from build123d import *

# Parameters (mm, degrees)
SKETCH2_W               = 58.32
SKETCH2_H               = 25.24
BOSS_EXTRUDE1_DEPTH     = 5
SKETCH1_R               = 2.25
SKETCH1_R_2             = 2.250000002
SKETCH1_R_3             = 2.250018527
CUT_EXTRUDE1_DEPTH      = 6
CUT_EXTRUDE1_DEPTH_BACK = 6
SKETCH3_W               = 42.063996433
SKETCH3_H               = 21.40000003
CUT_EXTRUDE2_DEPTH      = 1
CUT_EXTRUDE2_DEPTH_BACK = 11
SKETCH4_W               = 6.47
SKETCH4_H               = 0.8
CUT_EXTRUDE3_DEPTH      = 7.62


with BuildPart() as part:
    # Sketch2 → Boss-Extrude1 (new body, symmetric)
    with BuildSketch(Plane.XY):
        with Locations((50.422024802, 33.939282453)):
            Rectangle(SKETCH2_W, SKETCH2_H)
    extrude(amount=BOSS_EXTRUDE1_DEPTH, both=True)

    # Sketch1 → Cut-Extrude1 (cut, two sides)
    with BuildSketch(Plane.XY) as cut_extrude1_sk:
        with Locations((25.072024802, 28.939282453)):
            Circle(SKETCH1_R)
        with Locations((25.072024802, 38.939282453)):
            Circle(SKETCH1_R_2)
        with Locations((75.772021235, 38.939264272)):
            Circle(SKETCH1_R_3)
        with Locations((75.772024802, 28.939282453)):
            Circle(SKETCH1_R)
    extrude(amount=CUT_EXTRUDE1_DEPTH, mode=Mode.SUBTRACT)
    extrude(cut_extrude1_sk.sketch, amount=-CUT_EXTRUDE1_DEPTH_BACK, mode=Mode.SUBTRACT)

    # Sketch3 → Cut-Extrude2 (cut, two sides)
    with BuildSketch(Plane.XY.offset(5)) as cut_extrude2_sk:
        with Locations((50.422023018, 33.939282438)):
            Rectangle(SKETCH3_W, SKETCH3_H)
    extrude(amount=CUT_EXTRUDE2_DEPTH, mode=Mode.SUBTRACT)
    extrude(cut_extrude2_sk.sketch, amount=-CUT_EXTRUDE2_DEPTH_BACK, mode=Mode.SUBTRACT)

    # Sketch4 → Cut-Extrude3 (cut)
    with BuildSketch(Plane(origin=(0, 0, 5), x_dir=(-1, 0, 0), z_dir=(0, 0, -1))):
        with Locations((-74.689021235, 33.939282453)):
            Rectangle(SKETCH4_W, SKETCH4_H)
        with Locations((-26.155024802, 33.939282453)):
            Rectangle(SKETCH4_W, SKETCH4_H)
    extrude(amount=CUT_EXTRUDE3_DEPTH, mode=Mode.SUBTRACT)


solid = part.part
Verification items for the finished model (mm, model axes). A direction names the side the tool comes from. Coordinates: 2 decimals unless noted, no trailing zeros. Order: outer loops, then holes, each group sorted by start corner. A loop starts at its lowest first (then second) coordinate and runs counter-clockwise, first axis right, second up.
1. Go/stop test with a flat-tipped pin: pin 1 Ø5 at (x, y) = (25.07, 28.94) entering from -Z. Record where the tip stops, or that it passes through.
Results found:
pin 1: stops at z = -5
2. Sectioned sample at C-C, the plane z = 1.25. Record the cut outline in (x, y).
Results found:
outline: (21.26, 21.32) - (79.58, 21.32) - (79.58, 46.56) - (21.26, 46.56) - close; hole circle Ø4.5 at (25.07, 28.94); hole circle Ø4.5 at (25.07, 38.94); hole (22.92, 33.54) - (29.39, 33.54) - (29.39, 23.24) - (71.45, 23.24) - (71.45, 33.54) - (77.92, 33.54) - (77.92, 34.34) - (71.45, 34.34) - (71.45, 44.64) - (29.39, 44.64) - (29.39, 34.34) - (22.92, 34.34) - close; hole circle Ø4.5 at (75.77, 28.94); hole circle Ø4.5 at (75.77, 38.94)
3. Scan lines: line 1 (Y direction, x = 25, z = 1.25); line 2 (X direction, y = 35.5, z = 4); line 3 (Y direction, x = 44.5, z = -2). Record each from-to range of solid material in increasing order.
Results found:
line 1: y = 21.32 to 26.69, 31.19 to 33.54, 34.34 to 36.69, 41.19 to 46.56
line 2: x = 21.26 to 29.39, 71.45 to 79.58
line 3: y = 21.32 to 23.24, 44.64 to 46.56
4. Sectioned sample at A-A, the plane y = 24.75. Record the cut outline in (x, z).
Results found:
outline: (21.26, -5) - (29.39, -5) - (29.39, 5) - (21.26, 5) - close; (71.45, -5) - (79.58, -5) - (79.58, 5) - (71.45, 5) - close
5. Release check for a two-part mould opening along X. For faces 4 (the face through (50, 46.559, 0)), 5 (the face through (21.262, 34, 0)), 6 (the face through (24.584, 36.743, 0.07)), 7 (the face through (76.982, 30.836, 0.07)) record: +X half, -X half, draft (parallel to the pull), parting line (faces both ways), or undercut.
Results found:
face 4: draft
face 5: -X half
face 6: undercut
face 7: undercut
6. Set-up check for faces 1 (the face through (50, 23.239, 0)), 2 (the face through (75, 34.339, 1)), 3 (the face through (48, 23, 5)): record each of +Z, -Z, +X, -X, +Y, -Y from which the full face is reachable in a straight line by a thin tool's end or side.
Results found:
face 1: +Z, -Z
face 2: +Z
face 3: +Z, +X, -X, +Y, -Y
7. Sectioned sample at D-D, the plane y = 30. Record the cut outline in (x, z).
Results found:
outline: (21.26, -5) - (23.09, -5) - (23.09, 5) - (21.26, 5) - close; (27.06, -5) - (29.39, -5) - (29.39, 5) - (27.06, 5) - close; (71.45, -5) - (73.79, -5) - (73.79, 5) - (71.45, 5) - close; (77.76, -5) - (79.58, -5) - (79.58, 5) - (77.76, 5) - close
8. Sectioned sample at B-B, the plane x = 70.5. Record the cut outline in (y, z).
Results found:
outline: (21.32, -5) - (23.24, -5) - (23.24, 5) - (21.32, 5) - close; (44.64, -5) - (46.56, -5) - (46.56, 5) - (44.64, 5) - close
